Geometry check sheet. Reference: the model listing, model coordinates, mm. A direction names the side the tool comes from. Round coordinates to 2 decimals unless told otherwise and drop trailing zeros. Loops run counter-clockwise (first coordinate to the right, second up) from the corner with the lowest first, then second, coordinate; pieces in that order, holes last.
```python
from build123d import *

# Parameters (mm, degrees)
F0_R      = 50.8
F1_DEPTH  = 63.5
F2_R      = 44.45
F3_DEPTH  = 55.88
F4_R      = 44.45
F5_DEPTH  = 2.54
F6_SIZE   = 2.54
F8_R      = 16.51
F8_R_2    = 12.7
F9_DEPTH  = 50.8
F11_DEPTH = 44.45


# Not quite as in the source:
# - a fillet or chamfer that OpenCascade refuses, or shapes differently, is made with other operations: its cross-section is extruded or revolved along the edge and cut away or added


with BuildPart() as f1:
    # F0 (on Top) → F1 (new body)
    with BuildSketch(Plane.XY):
        Circle(F0_R)
    extrude(amount=F1_DEPTH)

    # F2 (on face) → F3 (cut)
    with BuildSketch(Plane.XY.offset(63.5)):
        Circle(F2_R)
    extrude(amount=-F3_DEPTH, mode=Mode.SUBTRACT)

    # F4 (on face) → F5 (cut)
    with BuildSketch(Plane(origin=(0, 0, 0), x_dir=(1, 0, 0), z_dir=(0, 0, -1))):
        Circle(F4_R)
    extrude(amount=-F5_DEPTH, mode=Mode.SUBTRACT)

    # F6
    f6_edges = [f1.edges().sort_by_distance(p)[0] for p in [
        (-50.8, 0, 63.5),
    ]]
    chamfer(f6_edges, length=F6_SIZE)

    # F7: fillet of radius 10.16 on 1 edges, made by hand

    # F7_s1 → F7_t2 (revolve, cut)
    with BuildSketch(Plane.XZ):
        with BuildLine():
            ThreePointArc((50.8, 56.7797916699), (50.1438097624, 60.3718941183), (48.26, 63.5))
            Line((48.26, 63.5), (50.8, 60.96))
            Line((50.8, 60.96), (50.8, 56.7797916699))
        make_face()
    revolve(axis=Axis((0, 0, 60.96), (0, 0, 1)), mode=Mode.SUBTRACT)

    # F8 (on face) → F9 (join)
    with BuildSketch(Plane.XY.offset(7.62)):
        Circle(F8_R)
        Circle(F8_R_2, mode=Mode.SUBTRACT)
    extrude(amount=F9_DEPTH)

    # F10 (on face) → F11 (cut)
    with BuildSketch(Plane.XY.offset(58.42)):
        with BuildLine():
            ThreePointArc((12.4434078933, 2.54), (12.6356891432, 1.2764638175), (12.7, 0))
            Line((12.7, 0), (14.605, 0))
            Line((14.605, 0), (14.605, 2.54))
            Line((14.605, 2.54), (12.4434078933, 2.54))
        make_face()
        with BuildLine():
            Line((14.605, 2.54), (14.605, 0))
            Line((14.605, 0), (16.51, 0))
            ThreePointArc((16.51, 0), (16.4607879997, 1.2737968559), (16.3134453749, 2.54))
            Line((16.3134453749, 2.54), (14.605, 2.54))
        make_face()
        with BuildLine():
            Line((16.51, 0), (14.605, 0))
            Line((14.605, 0), (14.605, -2.54))
            Line((14.605, -2.54), (16.3134453749, -2.54))
            ThreePointArc((16.3134453749, -2.54), (16.4607879997, -1.2737968559), (16.51, 0))
        make_face()
        with BuildLine():
            Line((14.605, 0), (12.7, 0))
            ThreePointArc((12.7, 0), (12.6356891432, -1.2764638175), (12.4434078933, -2.54))
            Line((12.4434078933, -2.54), (14.605, -2.54))
            Line((14.605, -2.54), (14.605, 0))
        make_face()
    extrude(amount=-F11_DEPTH, mode=Mode.SUBTRACT)


solid = f1.part
```
1) Mould release check, pull along X, two halves, no side actions. Record for faces 1 (the face through (0, -45, 0)), 2 (the face through (-12, -5, 58.42)), 3 (the face through (-11.012, -49.592, 27.992)): +X half, -X half, draft (parallel to the pull), parting line (faces both ways), or undercut.
Report:
face 1: draft
face 2: undercut
face 3: parting line
2) Sectioned sample at C-C, the plane y = 0. Record the cut outline in (x, z), then the cut area to 3 significant figures.
Report:
outline: (-50.8, 0) - (-44.45, 0) - (-44.45, 2.54) - (44.45, 2.54) - (44.45, 0) - (50.8, 0) - (50.8, 56.78) arc R10.16 ccw to (48.26, 63.5) - (44.45, 63.5) - (44.45, 7.62) - (16.51, 7.62) - (16.51, 13.97) - (12.7, 13.97) - (12.7, 7.62) - (-12.7, 7.62) - (-12.7, 58.42) - (-16.51, 58.42) - (-16.51, 7.62) - (-44.45, 7.62) - (-44.45, 63.5) - (-48.26, 63.5) arc R10.16 ccw to (-50.8, 56.78) - close
area: 1,470 mm2
3) Sectioned sample at A-A, the plane z = 23.5. Record the cut outline in (x, y), then the cut area to 3 significant figures.
Report:
outline: circle Ø101.6 at (0, 0); (12.44, -2.54) arc R12.7 cw (long way) to (12.44, 2.54) - (16.31, 2.54) arc R16.51 ccw (long way) to (16.31, -2.54) - close; hole circle Ø88.9 at (0, 0)
area: 2,230 mm2
4) Access from +Z, -Z, +X, -X, +Y, -Y to the whole of each face (thin tool, end or side, straight path). Record for faces 4 (the face through (42.397, 13.352, 35.951)), 5 (the face through (42.397, -13.352, 1.252)), 6 (the face through (14, -43, 63.5)).
Report:
face 4: +Z
face 5: -Z
face 6: +Z, +X, -X, +Y, -Y
5) Scan lines: line 1 along Y through (x, z) = (0, 20); line 2 along Y through (x, z) = (0, 0.85); line 3 along X through (y, z) = (11, 34). Record each from-to range of solid material in increasing order.
Report:
line 1: y = -50.8 to -44.45, -16.51 to -12.7, 12.7 to 16.51, 44.45 to 50.8
line 2: y = -50.8 to -44.45, 44.45 to 50.8
line 3: x = -49.59 to -43.07, -12.31 to -6.35, 6.35 to 12.31, 43.07 to 49.59
6) Gauge pin test, flat ends, axial feed: pin 1 (4 mm diameter, centred on y = 6, z = 48.5, fed in from -X); pin 2 (1.5 mm diameter, centred on x = -19, z = 56.5, fed in from -Y); pin 3 (20.5 mm diameter, centred on x = 2, y = 6, fed in from +Z). Record the tip position at first contact, or that the pin passes through.
Report:
pin 1: stops at x = -50.64
pin 2: stops at y = -47.41
pin 3: stops at z = 58.42
7) Sectioned sample at B-B, the plane x = 0. Record the cut outline in (y, z).
Report:
outline: (-50.8, 0) - (-44.45, 0) - (-44.45, 2.54) - (44.45, 2.54) - (44.45, 0) - (50.8, 0) - (50.8, 56.78) arc R10.16 ccw to (48.26, 63.5) - (44.45, 63.5) - (44.45, 7.62) - (16.51, 7.62) - (16.51, 58.42) - (12.7, 58.42) - (12.7, 7.62) - (-12.7, 7.62) - (-12.7, 58.42) - (-16.51, 58.42) - (-16.51, 7.62) - (-44.45, 7.62) - (-44.45, 63.5) - (-48.26, 63.5) arc R10.16 ccw to (-50.8, 56.78) - close
